The drawing under review shows one solid part. Ordinate dimensions are in mm from its lowest x, y, z. A direction names the side the tool comes from. Coordinates: 2 decimals unless noted, no trailing zeros. Write each loop counter-clockwise with the first axis right and the second up, starting at its lowest first coordinate (ties: lowest second). Pieces come first, ordered by that corner, then holes.
1) We need section B-B on y = 4.25. Write out the cut boundary in (x, z).
2) We need section D-D on z = 25.25. Write out the cut boundary in (x, y) (1 decimal).
3) We need section C-C on z = 15.5. Give the number of separate pieces and of enclosed holes in the cut face, then the cut area to 3 significant figures.
4) We need section A-A on x = 14. Write out the cut boundary in (y, z) (1 decimal).
5) For the marked faces 1, 2, 3, 4 and 5, list the 3-axis set-ups (+Z, -Z, +X, -X, +Y, -Y) from which the entire face can be reached by the end or side of a thin tool; tool diameter is ignored.
6) Insertion check: P1, Ø2.5, axis at x = 29.36, y = 1.56, coming from the +Z side; P2, Ø5, axis at x = 22.5, z = 17, coming from the -Y side (1 decimal); P3, Ø2.5, axis at y = 19, z = 1, coming from the -X side; P4, Ø7, axis at x = 14.5, y = 13, coming from the +Z side. Each pin has a flat end and moves straight along its axis. Give the tip position at first contact, or say it passes through.
7) To check wall thickness, follow line 1 along Z through (x, y) = (51, 6); line 2 along X through (y, z) = (1, 15.75) (1 decimal); line 3 along Z through (x, y) = (19.5, 9.25). State the ranges of each line that lie inside material, in increasing order.
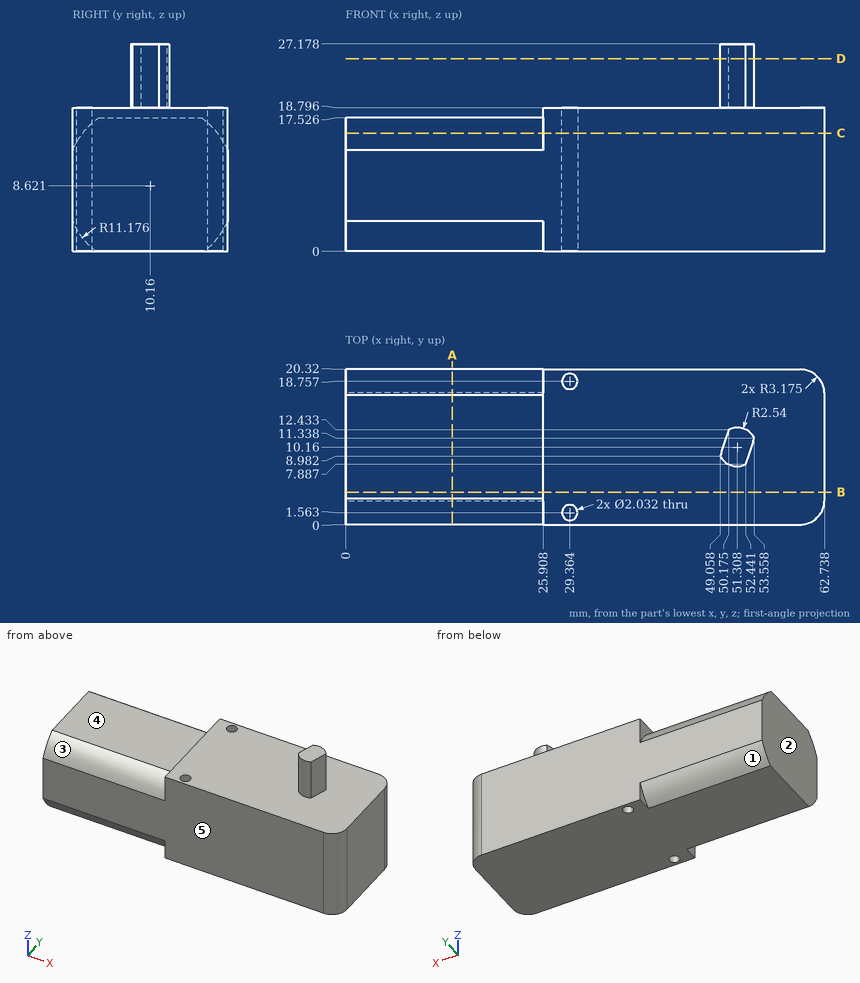
Result:
1. outline: (0, 0) - (62.74, 0) - (62.74, 18.8) - (25.91, 18.8) - (25.91, 17.53) - (0, 17.53) - close
2. outline: (49.1, 9) arc R2.5 ccw to (52.4, 7.9) - (53.6, 11.3) arc R2.5 ccw to (50.2, 12.4) - close
3. separate pieces: 1
3. enclosed holes: 2
3. area: 1,190 mm2
4. outline: (0, 4) arc R11.2 ccw to (3, 0) - (17.3, 0) arc R11.2 ccw to (20.3, 4) - (20.3, 13.3) arc R11.2 ccw to (16.9, 17.5) - (3.4, 17.5) arc R11.2 ccw to (0, 13.3) - close
5. face 1: -Z, -X, +Y
5. face 2: +Z, -Z, -X, +Y, -Y
5. face 3: +Z, -X, -Y
5. face 4: +Z, -X, +Y, -Y
5. face 5: +Z, -Z, +X, -X, -Y
6. P1: stops at z = 18.8
6. P2: stops at y = 0.7
6. P3: stops at x = 0
6. P4: stops at z = 17.53
7. line 1: z = 0 to 18.8
7. line 2: x = 25.9 to 28.5, 30.2 to 61.9
7. line 3: z = 0 to 17.53
